```python
from build123d import *

# Parameters (mm, degrees)
AUFSATZ_LINEAR_AUSTRAGEN1_DEPTH = 4
AUFSATZ_LINEAR_START            = 20
AUFSATZ_LINEAR_AUSTRAGEN2_DEPTH = 20
VERRUNDUNG1_R                   = 20


with BuildPart() as part:
    # Skizze1 → Aufsatz-Linear austragen1 (new body)
    with BuildSketch(Plane(origin=(0, 0, 0), x_dir=(1, 0, 0), z_dir=(0, 1, 0))):
        with BuildLine():
            Line((-10, 69.282032303), (-10, -69.282032303))
            ThreePointArc((-10, -69.282032303), (0, -70), (10, -69.282032303))
            Line((10, -69.282032303), (10, 69.282032303))
            ThreePointArc((10, 69.282032303), (0, 70), (-10, 69.282032303))
        make_face()
    extrude(amount=AUFSATZ_LINEAR_AUSTRAGEN1_DEPTH)

    # Skizze2 → Aufsatz-Linear austragen2 (add)
    with BuildSketch(Plane.XZ.offset(AUFSATZ_LINEAR_START)):
        with BuildLine():
            Line((-10, 69.282032303), (-10, 64.282032303))
            ThreePointArc((-10, 64.282032303), (0, 65.055204842), (10, 64.282032303))
            Line((10, 64.282032303), (10, 69.282032303))
            ThreePointArc((10, 69.282032303), (0, 70), (-10, 69.282032303))
        make_face()
        with BuildLine():
            Line((-10, -64.282032303), (-10, -69.282032303))
            ThreePointArc((-10, -69.282032303), (0, -70), (10, -69.282032303))
            Line((10, -69.282032303), (10, -64.282032303))
            ThreePointArc((10, -64.282032303), (0, -65.055204842), (-10, -64.282032303))
        make_face()
    extrude(amount=-AUFSATZ_LINEAR_AUSTRAGEN2_DEPTH)

    # Verrundung1
    verrundung1_edges = [part.edges().sort_by_distance(p)[0] for p in [
        (0, 0, 65.055204842),
        (0, 0, -65.055204842),
    ]]
    fillet(verrundung1_edges, radius=VERRUNDUNG1_R - 0.0001)  # a hair under: the kernel refuses the full size


solid = part.part
```
The listing builds one solid part. Answer for the finished solid, in the listing's coordinates (mm). Coordinates: 2 decimals unless noted, no trailing zeros. Loops run counter-clockwise (first coordinate to the right, second up) from the corner with the lowest first, then second, coordinate; pieces in that order, holes last. Notation, with made-up numbers: (46, -1.75) -> (55, -1.75) arc R11 cw to (55, 15.25) -> close; hole circle Ø11 at (26, -39.5). An arc over 180 degrees is marked (long way). Use one line per item in the form item = value. Start each with the question number.
Item 1: The part is cut by section A-A on y = -8. Determine the outline of the cut face in (x, z).
Item 2: Consider L1, parallel to Y at x = 8.5, z = 14; L2, parallel to Z at x = 6.25, y = -7; L3, parallel to Z at x = -9, y = -12. Determine where each line is inside the solid, lowest interval first. Write a range as [from, to].
Item 3: The part is cut by section B-B on z = 1.5. Determine the outline of the cut face in (x, y).
Item 4: The mould has two halves that part along Z. Classify faces 1 (the face through (0, -20, -67)), 2 (the face through (0, -8, -70)), 3 (the face through (0, 0, -1)), 4 (the face through (0, -8, 70)): released by +Z, released by -Z, zero draft, split by the parting line, or undercut.
Item 5: Flat-ended cylindrical pins translate along their axes: pin 1 Ø8 at (y, z) = (-6, -0.5) entering from +X; pin 2 Ø10 at (x, z) = (2, -5) entering from -Y; pin 3 Ø5 at (x, y) = (-7, -6.5) entering from +Z. Find the tip coordinate at first contact, or state that the pin passes through.
Answer key:
q1.outline = (-10, -69.28) arc R70 ccw to (10, -69.28) -> (10, -60.23) arc R61.06 cw to (-10, -60.23) -> close; (-10, 60.23) arc R61.06 cw to (10, 60.23) -> (10, 69.28) arc R70 ccw to (-10, 69.28) -> close
q2.L1 = [0, 4]
q2.L2 = [-69.72, -59.93], [59.93, 69.72]
q2.L3 = [-69.42, -62.74], [62.74, 69.42]
q3.outline = (-10, 0) -> (10, 0) -> (10, 4) -> (-10, 4) -> close
q4.face_1 = zero draft
q4.face_2 = released by -Z
q4.face_3 = undercut
q4.face_4 = released by +Z
q5.pin_1 = through
q5.pin_2 = 0
q5.pin_3 = 69.86
